Design review of the part shown in the three views and the two pictorial views. Dimensions are in mm from the part's minimum x, y and z. Round coordinates to 2 decimals unless told otherwise and drop trailing zeros. Order: outer loops, then holes, each group sorted by start corner. A loop starts at its lowest first (then second) coordinate and runs counter-clockwise, first axis right, second up.
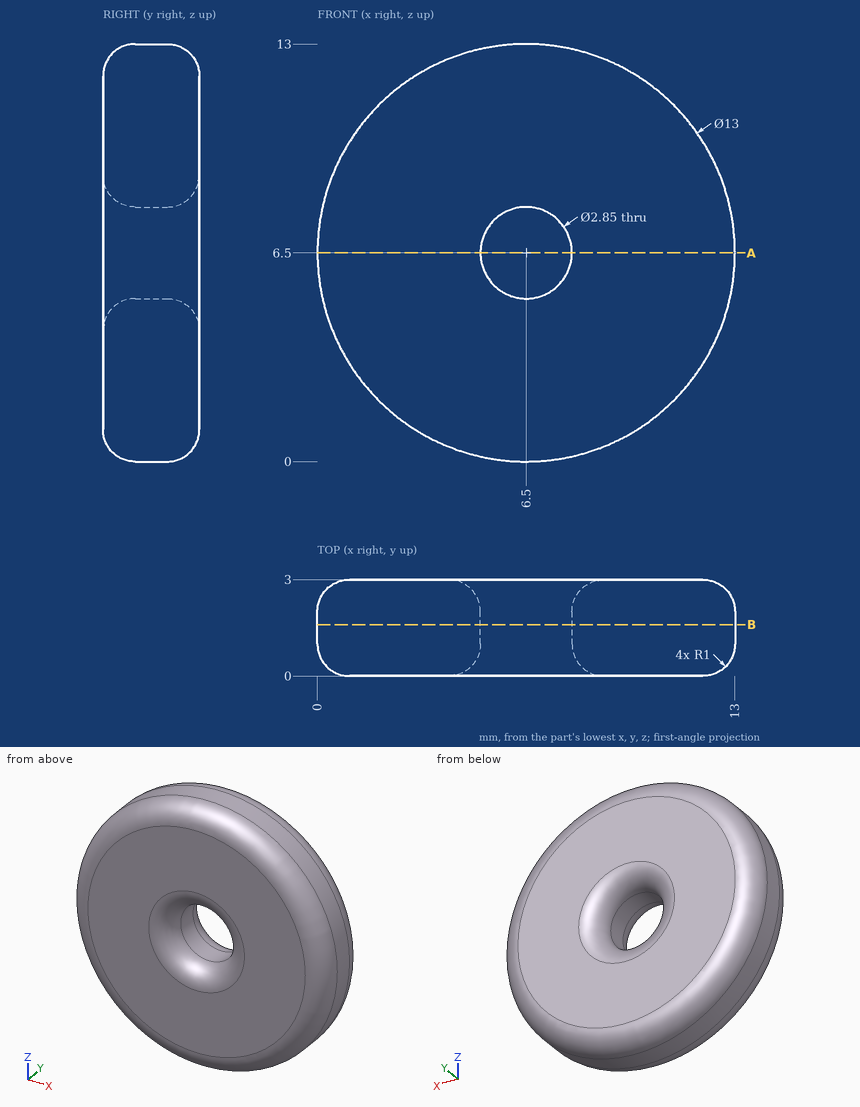
1) To check wall thickness, follow line 1 along Z through (x, y) = (6.5, 1.65) (3 decimals); line 2 along Z through (x, y) = (6, 1.8). State the ranges of each line that lie inside material, in increasing order.
Results:
line 1: z = 0 to 5.075, 7.925 to 13
line 2: z = 0.02 to 5.17, 7.83 to 12.98
2) Clearance check with flat-ended pins moving along their axes: P1, Ø4, axis at x = 6.5, z = 6.5, coming from the +Y side; P2, Ø4.5, axis at x = 6.5, z = 6.5, coming from the -Y side; P3, Ø1, axis at x = 5.5, y = 1, coming from the -Z side. State where each tip first meets the part, or that it passes through.
Results:
P1: stops at y = 2.91
P2: stops at y = 0.02
P3: stops at z = 0.02
3) Take a section at A-A on z = 6.5. Give the boundary of the cut face in (x, y) (3 decimals), plus the area to 3 significant figures.
Results:
outline: (0, 1) arc R1 ccw to (1, 0) - (4.075, 0) arc R1 ccw to (5.075, 1) - (5.075, 2) arc R1 ccw to (4.075, 3) - (1, 3) arc R1 ccw to (0, 2) - close; (7.925, 1) arc R1 ccw to (8.925, 0) - (12, 0) arc R1 ccw to (13, 1) - (13, 2) arc R1 ccw to (12, 3) - (8.925, 3) arc R1 ccw to (7.925, 2) - close
area: 28.7 mm2
4) Take a section at B-B on y = 1.6. Give the boundary of the cut face in (x, z) (3 decimals), plus the area to 3 significant figures.
Results:
outline: circle Ø13 at (6.5, 6.5); hole circle Ø2.85 at (6.5, 6.5)
area: 126 mm2
